Autodesk Inventor part; units mm, degrees
ref_plane "Work Plane2" through (0, 10, 0) normal (0, 1, 0) x (1, 0, 0)
ref_plane "YZ Plane" through (0, 0, 0) normal (1, 0, 0) x (0, 1, 0)
ref_plane "XZ Plane" through (0, 0, 0) normal (0, 1, 0) x (-1, 0, 0)
sketch "Sketch1" plane through (0, 0, 0) normal (0, 1, 0) x (-1, 0, 0)
  circle A0 centre (0, 0) radius 74.5
  circle A1 centre (0, 0) radius 69.5
  circle A2 centre (0, 0) radius 66.5
  dimension "Absolute_Diameter" = 149
  dimension "Diameter_No_Outer_Lip" = 139
  dimension "Inner_Cylinder_Diameter" = 133
extrude "Extrusion1" add sketch "Sketch1" along normal blind 4 contours A0
extrude "Extrusion2" add sketch "Sketch1" along normal blind 60 contours A1
sketch "Sketch2" plane through (0, 60, 0) normal (0, 1, 0) x (1, 0, 0)
  circle A0 centre (0, 0) radius 61.5
  circle A1 centre (0, 0) radius 66.5
  dimension "Lip_Diameter_Out" = 123
  dimension "Top_Outer_Lip_Diameter" = 133
extrude "Extrusion7" add sketch "Sketch2" against normal blind 4
ref_plane "Work Plane2" through (0, 10, 0) normal (0, 1, 0) x (1, 0, 0)
sketch "Sketch3" plane through (0, 10, 0) normal (0, 1, 0) x (1, 0, 0)
  circle A0 centre (0, 0) radius 127.5
  circle A1 centre (-127.5, 0) radius 2.5
  circle A2 centre (-103.1497, -74.9426) radius 2.5
  circle A3 centre (-39.3997, -121.2597) radius 2.5
  circle A4 centre (39.3997, -121.2597) radius 2.5
  circle A5 centre (103.1497, -74.9426) radius 2.5
  circle A6 centre (127.5, 0) radius 2.5
  circle A7 centre (103.1497, 74.9426) radius 2.5
  circle A8 centre (39.3997, 121.2597) radius 2.5
  circle A9 centre (-39.3997, 121.2597) radius 2.5
  circle A10 centre (-103.1497, 74.9426) radius 2.5
  dimension "d27" = 255
  dimension "d28" = 5
  dimension "d31" = 360
extrude "Extrusion8" [suppressed]
sketch "Sketch24" plane through (0, 60, 0) normal (0, 1, 0) x (1, 0, 0)
  circle A0 centre (0, 0) radius 51
  circle A1 centre (0, -51) radius 2.75
  circle A2 centre (44.1673, -25.5) radius 2.75
  circle A3 centre (44.1673, 25.5) radius 2.75
  circle A4 centre (0, 51) radius 2.75
  circle A5 centre (-44.1673, 25.5) radius 2.75
  circle A6 centre (-44.1673, -25.5) radius 2.75
  dimension "d230" = 102
  dimension "d231" = 5.5
  dimension "d234" = 360
extrude "Extrusion30" [suppressed]
sketch "Sketch25" plane through (0, 60, 0) normal (0, 1, 0) x (1, 0, 0)
  point P0 (0, 0)
sketch "Sketch26" plane through (0, 60, 0) normal (0, 1, 0) x (1, 0, 0)
  circle A0 centre (-44.1673, 25.5) radius 2.75
  circle A1 centre (0, 0) radius 51
  circle A2 centre (-51, 0) radius 3.25
  circle A3 centre (-25.5, -44.1673) radius 3.25
  circle A4 centre (25.5, -44.1673) radius 3.25
  circle A5 centre (51, 0) radius 3.25
  circle A6 centre (25.5, 44.1673) radius 3.25
  circle A7 centre (-25.5, 44.1673) radius 3.25
  dimension "d239" = 6.5
  dimension "d242" = 360
extrude "Extrusion31" [suppressed]
properties part number "Cylinder Replacement- 10"
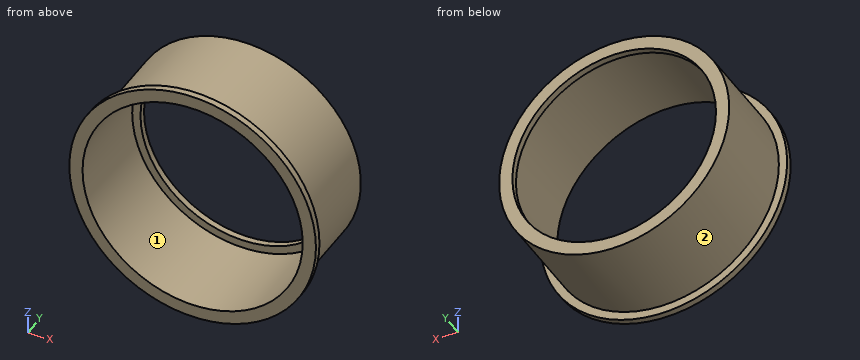
Can you work these out from the model? Positions are in its coordinate system, mm. Face numbers are marked on the shaded views. Give positions to 0.01 mm unless a question says otherwise; leave off trailing zeros. Order: outer loops, then holes, each group sorted by start corner. A loop starts at its lowest first (then second) coordinate and runs counter-clockwise, first axis right, second up. Notation, with made-up numbers: M -21.5,-33.5 L 16.5,-33.5 A18 cw 16.5,-8.5 Z; hole C -23.5,-31.5 d9. An arc over 180 degrees is marked long. Use one line per item in the form item = value. Start each with the question number.
Item 1: We'd pull the mould along Z, two halves only. Please class the marked faces 1 and 2: +Z half, -Z half, draft (parallel to the pull), parting line (faces both ways), or undercut.
Item 2: If we section it at A-A (x = 0): Write out the boundary of the cut face in (y, z), then the cut area to 3 significant figures.
Item 3: If we section it at B-B (z = 0): Write out the boundary of the cut face in (x, y).
Item 4: Will these pins go through, and if not, where does the flat tip stop? pin 1 Ø8 at (x, z) = (13.5, -57) entering from -Y; pin 2 Ø2 at (x, y) = (37.5, 34) entering from +Z; pin 3 Ø5 at (y, z) = (42, -1.5) entering from -X.
Item 5: If I drill on line 1 along Z through (x, y) = (0, 19); line 2 along Z through (x, y) = (0, 57.5); line 3 along X through (y, z) = (37, 52.5), over which ranges is the centre line in solid material (lowest first)?
Item 6: If we section it at C-C (y = 19): Write out the boundary of the cut face in (x, z), then the cut area to 3 significant figures.
Outcome:
q1.face_1 = undercut
q1.face_2 = parting line
q2.outline = M 0,-74.5 L 4,-74.5 L 4,-69.5 L 60,-69.5 L 60,-61.5 L 56,-61.5 L 56,-66.5 L 0,-66.5 Z; M 0,66.5 L 56,66.5 L 56,61.5 L 60,61.5 L 60,69.5 L 4,69.5 L 4,74.5 L 0,74.5 Z
q2.area = 440 mm2
q3.outline = M -74.5,0 L -66.5,0 L -66.5,56 L -61.5,56 L -61.5,60 L -69.5,60 L -69.5,4 L -74.5,4 Z; M 61.5,56 L 66.5,56 L 66.5,0 L 74.5,0 L 74.5,4 L 69.5,4 L 69.5,60 L 61.5,60 Z
q4.pin_1 = 56
q4.pin_2 = 59.14
q4.pin_3 = -69.5
q5.line_1 = -69.5 to -66.5, 66.5 to 69.5
q5.line_2 = -69.5 to -61.5, 61.5 to 69.5
q5.line_3 = -45.54 to -40.82, 40.82 to 45.54
q6.outline = C 0,0 d139; hole C 0,0 d133
q6.area = 1,280 mm2
